Here's how the part is built. I have some questions about the finished solid (model axes, mm). Give positions to 0.01 mm unless a question says otherwise; leave off trailing zeros. Write each loop counter-clockwise with the first axis right and the second up, starting at its lowest first coordinate (ties: lowest second). Pieces come first, ordered by that corner, then holes. Notation, with made-up numbers: (6.25, 82.5) -> (30.25, 82.5) arc R26 cw to (30.25, 116.5) -> close; hole circle Ø7 at (35, 14). An arc over 180 degrees is marked (long way). Put each result on its own line as item: value. Start each with the question number.
from build123d import *

# Parameters (mm, degrees)
SKETCH1_R                  = 200.533
SKETCH1_R_2                = 104.775
BOSS_EXTRUDE1_DEPTH        = 6.35
F_9_0_196_DIAMETER_HOLE1_D = 4.9784


with BuildPart() as part:
    # Sketch1 → Boss-Extrude1 (new body)
    with BuildSketch(Plane(origin=(0, 0, 0), x_dir=(0, 1, 0), z_dir=(0, 0, 1))):
        with Locations(Location((0, 0, 0), (0, 0, 270))):
            Circle(SKETCH1_R)
        with Locations(Location((0, 0, 0), (0, 0, 270))):
            Circle(SKETCH1_R_2, mode=Mode.SUBTRACT)
    extrude(amount=BOSS_EXTRUDE1_DEPTH)

    # #9 (0.196) Diameter Hole1 (through all)
    with Locations(Plane.XY.offset(6.35)):
        with Locations((-96.774, 167.617484852), (-167.617484852, 96.774), (-193.548, 0), (-167.617484852, -96.774), (-96.774, -167.617484852), (0, -193.548), (96.774, -167.617484852), (167.617484852, -96.774), (193.548, 0), (167.617484852, 96.774), (96.774, 167.617484852), (0, 193.548)):
            Hole(F_9_0_196_DIAMETER_HOLE1_D / 2)


solid = part.part
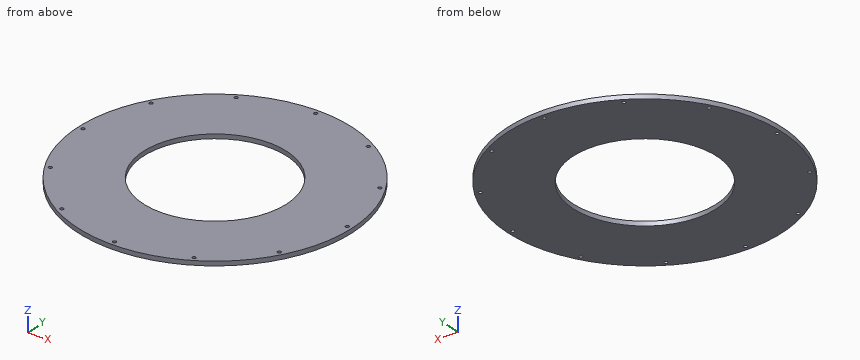
1) I want a section at B-B, the plane y = 65.5. Write out the boundary of the cut face in (x, z), and give its area (3 significant figures).
2) I'm going to push flat-ended pins straight in: pin 1 Ø1.5 at (x, z) = (54.5, 2) entering from -Y; pin 2 Ø1 at (y, z) = (-148.5, 1) entering from -X; pin 3 Ø3 at (x, z) = (14.5, 3) entering from +Y. Where does each tip first touch, or does it pass through?
3) I want a section at A-A, the plane x = 85. Write out the boundary of the cut face in (y, z), and give its area (3 significant figures).
4) I need wall thicknesses on probe 1 along Y at (x, z) = (167.5, 2.75); probe 2 along X at (y, z) = (-3, 5); probe 3 along X at (y, z) = (36.5, 1.5). Which ranges of each line are inside material? Lowest first, please.
5) I want a section at D-D, the plane x = -116.5. Write out the boundary of the cut face in (y, z).
6) I want a section at C-C, the plane z = 1.5. State how many separate pieces and enclosed holes the cut face has, and give its area (3 significant figures).
Established:
1. outline: (-189.53, 0) -> (-81.78, 0) -> (-81.78, 6.35) -> (-189.53, 6.35) -> close; (81.78, 0) -> (189.53, 0) -> (189.53, 6.35) -> (81.78, 6.35) -> close
1. area: 1,370 mm2
2. pin 1: stops at y = -193.2
2. pin 2: stops at x = -135.31
2. pin 3: stops at y = 200.11
3. outline: (-181.63, 0) -> (-61.26, 0) -> (-61.26, 6.35) -> (-181.63, 6.35) -> close; (61.26, 0) -> (181.63, 0) -> (181.63, 6.35) -> (61.26, 6.35) -> close
3. area: 1,530 mm2
4. probe 1: y = -110.26 to -99.26, -94.29 to 94.29, 99.26 to 110.26
4. probe 2: x = -200.51 to -104.73, 104.73 to 200.51
4. probe 3: x = -197.18 to -98.21, 98.21 to 197.18
5. outline: (-163.22, 0) -> (163.22, 0) -> (163.22, 6.35) -> (-163.22, 6.35) -> close
6. separate pieces: 1
6. enclosed holes: 13
6. area: 91,600 mm2
